Design review of the part built by this model. Coordinates are the model's own, in mm. Face numbers are marked on the shaded views. A direction names the side the tool comes from. Coordinates: 2 decimals unless noted, no trailing zeros. Write each loop counter-clockwise with the first axis right and the second up, starting at its lowest first coordinate (ties: lowest second). Pieces come first, ordered by that corner, then holes.
```python
from build123d import *

# Parameters (mm, degrees)
F0_W      = 40
F0_H      = 64
F1_DEPTH  = 3
F2_W      = 10
F2_H      = 64
F2_W_2    = 40
F3_DEPTH  = 3
F4_R      = 1.6
F5_DEPTH  = 25
F6_R      = 1.6
F7_DEPTH  = 25
F8_R      = 3.75
F9_DEPTH  = 3
F10_R     = 2
F11_DEPTH = 25


with BuildPart() as f1:
    # F0 (on Top) → F1 (new body)
    with BuildSketch(Plane.XY):
        Rectangle(F0_W, F0_H)
    extrude(amount=F1_DEPTH)

    # F2 (on face) → F3 (join)
    with BuildSketch(Plane.XY.offset(3)):
        with Locations((-25, 0)):
            Rectangle(F2_W, F2_H)
        Rectangle(F2_W_2, F2_H)
        with Locations((25, 0)):
            Rectangle(F2_W, F2_H)
    extrude(amount=F3_DEPTH)

    # F4 (on face) → F5 (cut)
    with BuildSketch(Plane.XY.offset(6)):
        with Locations((-25, 16.3)):
            Circle(F4_R)
    extrude(amount=-F5_DEPTH, mode=Mode.SUBTRACT)

    # F6 (on face) → F7 (cut)
    with BuildSketch(Plane.XY.offset(6)):
        with Locations((-25, -22)):
            Circle(F6_R)
        with Locations((25, -22)):
            Circle(F6_R)
        with Locations((25, 16.3)):
            Circle(F6_R)
    extrude(amount=-F7_DEPTH, mode=Mode.SUBTRACT)

    # F8 (on face) → F9 (cut)
    with BuildSketch(Plane.XY.offset(6)):
        with Locations((-10.2, -15)):
            Circle(F8_R)
        with Locations((10.2, -15)):
            Circle(F8_R)
        with Locations((10.2, 15)):
            Circle(F8_R)
        with Locations((-10.2, 15)):
            Circle(F8_R)
    extrude(amount=-F9_DEPTH, mode=Mode.SUBTRACT)

    # F10 (on face) → F11 (cut)
    with BuildSketch(Plane.XY.offset(3)):
        with Locations((-10.2, -15)):
            Circle(F10_R)
        with Locations((-10.2, 15)):
            Circle(F10_R)
        with Locations((10.2, 15)):
            Circle(F10_R)
        with Locations((10.2, -15)):
            Circle(F10_R)
    extrude(amount=-F11_DEPTH, mode=Mode.SUBTRACT)


solid = f1.part
```
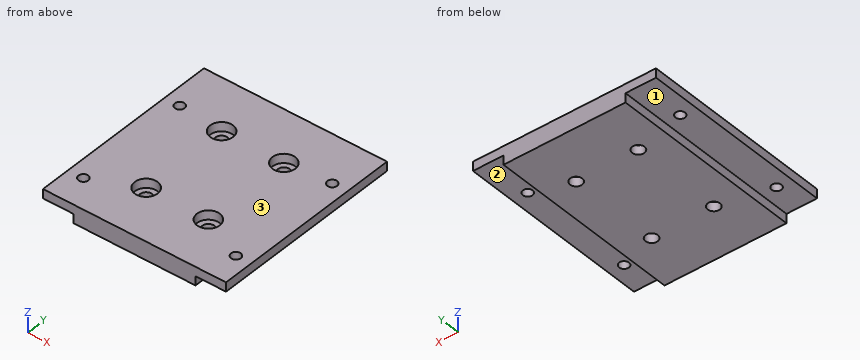
(1) Consider section D-D (y = -0.5). Give the boundary of the cut face in (x, z).
(2) Consider section B-B (y = -22). Give the boundary of the cut face in (x, z), plus the area to 3 significant figures.
(3) For the marked faces 1, 2 and 3, list the 3-axis set-ups (+Z, -Z, +X, -X, +Y, -Y) from which the entire face can be reached by the end or side of a thin tool; tool diameter is ignored.
(4) Wall thickness on line 1 (Y direction, x = 10.2, z = 2.3); line 2 (Y direction, x = -10.2, z = 4.1); line 3 (X direction, y = -15.5, z = 0.45): over which ranges is each line inside the solid? List them lowest first.
(5) Consider section C-C (z = 2.1). Give the boundary of the cut face in (x, y), plus the area to 3 significant figures.
(6) Insertion check: pin 1 Ø3 at (x, y) = (25, -22) entering from -Z; pin 2 Ø1.5 at (y, z) = (16, 1) entering from +X; pin 3 Ø2 at (x, y) = (-8.5, -15.5) entering from +Z; pin 4 Ø0.9 at (y, z) = (9, 1.5) entering from -X. Each pin has a flat end and moves straight along its axis. Give the tip position at first contact, or say it passes through.
(7) Consider section A-A (x = -25). Give the boundary of the cut face in (y, z).
Results:
1. outline: (-30, 3) - (-20, 3) - (-20, 0) - (20, 0) - (20, 3) - (30, 3) - (30, 6) - (-30, 6) - close
2. outline: (-30, 3) - (-26.6, 3) - (-26.6, 6) - (-30, 6) - close; (-23.4, 3) - (-20, 3) - (-20, 0) - (20, 0) - (20, 3) - (23.4, 3) - (23.4, 6) - (-23.4, 6) - close; (26.6, 3) - (30, 3) - (30, 6) - (26.6, 6) - close
2. area: 281 mm2
3. face 1: -Z, -X, +Y, -Y
3. face 2: -Z, +X, +Y, -Y
3. face 3: +Z, +X, -X, +Y, -Y
4. line 1: y = -32 to -17, -13 to 13, 17 to 32
4. line 2: y = -32 to -18.75, -11.25 to 11.25, 18.75 to 32
4. line 3: x = -20 to -12.14, -8.26 to 8.26, 12.14 to 20
5. outline: (-20, -32) - (20, -32) - (20, 32) - (-20, 32) - close; hole circle Ø4 at (-10.2, -15); hole circle Ø4 at (-10.2, 15); hole circle Ø4 at (10.2, -15); hole circle Ø4 at (10.2, 15)
5. area: 2,510 mm2
6. pin 1: passes through
6. pin 2: stops at x = 20
6. pin 3: stops at z = 3
6. pin 4: stops at x = -20
7. outline: (-32, 3) - (-23.6, 3) - (-23.6, 6) - (-32, 6) - close; (-20.4, 3) - (14.7, 3) - (14.7, 6) - (-20.4, 6) - close; (17.9, 3) - (32, 3) - (32, 6) - (17.9, 6) - close
